Work out the finished part from the listing and answer in its coordinate system (mm). Face numbers are marked on the shaded views. A direction names the side the tool comes from. Round coordinates to 2 decimals unless told otherwise and drop trailing zeros. Loops run counter-clockwise (first coordinate to the right, second up) from the corner with the lowest first, then second, coordinate; pieces in that order, holes last. Notation, with made-up numbers: (19, 58.25) - (25, 58.25) arc R28 cw to (25, 96.25) - close; hole circle Ø5 at (1, 70). An arc over 180 degrees is marked (long way). Return JSON: item names as keys, results as strings.
from build123d import *

# Parameters (mm, degrees)
F0_W     = 500
F0_H     = 350
F1_DEPTH = 500


with BuildPart() as f1:
    # F0 (on Right) → F1 (new body)
    with BuildSketch(Plane.YZ):
        Rectangle(F0_W, F0_H)
        Polygon((-450, -175), (-250, -175), (-250, 175), (-250, 725), (-450, 725), align=None)
    extrude(amount=F1_DEPTH)


solid = f1.part
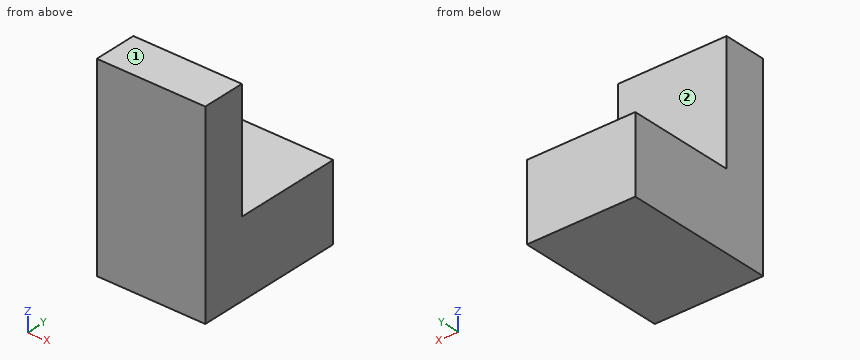
1) Section C-C (z = 576.5) is taken. Give the vertices of the cut face in (x, y).
Verdict:
{"outline": "(0, -450) - (500, -450) - (500, -250) - (0, -250) - close"}
2) Section A-A (x = 392.5) is taken. Give the vertices of the cut face in (y, z), and give its area (3 significant figures).
Verdict:
{"outline": "(-450, -175) - (250, -175) - (250, 175) - (-250, 175) - (-250, 725) - (-450, 725) - close", "area": "355,000 mm2"}
3) Flat-ended cylindrical pins translate along their axes: pin 1 (3 mm diameter, centred on x = 119.5, z = 443.5, fed in from +Y); pin 2 (12 mm diameter, centred on x = 307, y = -135, fed in from +Z). Find the tip coordinate at first contact, or state that the pin passes through.
Verdict:
{"pin 1": "stops at y = -250", "pin 2": "stops at z = 175"}
4) Section B-B (y = -192.5) is taken. Give the vertices of the cut face in (x, z), and give its area (3 significant figures).
Verdict:
{"outline": "(0, -175) - (500, -175) - (500, 175) - (0, 175) - close", "area": "175,000 mm2"}
5) A tool of negligible diameter and unlimited length cuts with its end or side. For the marked faces 1 and 2, from which of +Z, -Z, +X, -X, +Y, -Y can it reach the whole face along a straight path? Write none if from no direction.
Verdict:
{"face 1": "+Z, +X, -X, +Y, -Y", "face 2": "+Z, +X, -X, +Y"}
6) Find the intervals of material crossed by L1, parallel to Y at x = 434, z = 581.5; L2, parallel to Z at x = 44.5, y = -217, in increasing order.
Verdict:
{"L1": "y = -450 to -250", "L2": "z = -175 to 175"}
